Work out the finished part from the listing and answer in its coordinate system (mm). Face numbers are marked on the shaded views. A direction names the side the tool comes from. Round coordinates to 2 decimals unless told otherwise and drop trailing zeros. Loops run counter-clockwise (first coordinate to the right, second up) from the corner with the lowest first, then second, coordinate; pieces in that order, holes last. Notation, with made-up numbers: M -3.75,21.5 L 38.25,21.5 A17 ccw 38.25,41.5 Z; hole C 5,-10.5 d8. An arc over 180 degrees is marked long. One line per item, written item: value.
```python
from build123d import *

# Parameters (mm, degrees)
F0_W     = 76.2
F0_H     = 50.8
F0_R     = 12.7
F1_DEPTH = 12.7
F2_W     = 6.35
F2_H     = 50.8
F3_DEPTH = 2.54
F5_DEPTH = 50.801
F6_R     = 4.445
F7_DEPTH = 12.7


with BuildPart() as f1:
    # F0 (on Front) → F1 (new body)
    with BuildSketch(Plane.XZ):
        Rectangle(F0_W, F0_H)
        Circle(F0_R, mode=Mode.SUBTRACT)
    extrude(amount=F1_DEPTH)

    # F2 (on face) → F3 (cut)
    with BuildSketch(Plane.XZ.offset(12.7)):
        with Locations((-32.385, 0)):
            Rectangle(F2_W, F2_H)
        with BuildLine():
            Line((6.35, 25.4), (-6.35, 25.4))
            Line((-6.35, 25.4), (-6.35, 10.9985226281))
            ThreePointArc((-6.35, 10.9985226281), (0, 12.7), (6.35, 10.9985226281))
            Line((6.35, 10.9985226281), (6.35, 25.4))
        make_face()
        with BuildLine():
            Line((-6.35, -10.9985226281), (-6.35, -25.4))
            Line((-6.35, -25.4), (6.35, -25.4))
            Line((6.35, -25.4), (6.35, -10.9985226281))
            ThreePointArc((6.35, -10.9985226281), (0, -12.7), (-6.35, -10.9985226281))
        make_face()
    extrude(amount=-F3_DEPTH, mode=Mode.SUBTRACT)

    # F4 (on face) → F5 (cut, through all)
    with BuildSketch(Plane(origin=(0, 0, -25.4), x_dir=(1, 0, 0), z_dir=(0, 0, -1))):
        Polygon((31.75, 12.7), (19.05, 12.7), (16.1170606325, 7.62), (34.6829393675, 7.62), align=None)
    extrude(amount=-F5_DEPTH, mode=Mode.SUBTRACT)

    # F6 (on face) → F7 (join)
    with BuildSketch(Plane.YZ.offset(38.1)):
        with Locations((-6.35, 0)):
            Circle(F6_R)
    extrude(amount=F7_DEPTH)


solid = f1.part
```
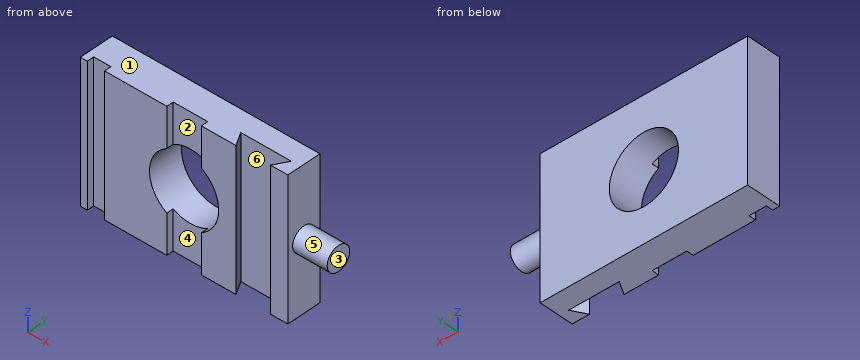
1) The mould has two halves that part along X. Classify the marked faces 3, 4, 5 and 6: +X half, -X half, draft (parallel to the pull), parting line (faces both ways), or undercut.
Check values:
face 3: +X half
face 4: undercut
face 5: draft
face 6: undercut
2) Find the intervals of material crossed by probe 1 along Z at (x, y) = (0, -10); probe 2 along X at (y, z) = (-4.75, 0); probe 3 along X at (y, z) = (-8.5, 1.5), in increasing order. Write a range as from..to.
Check values:
probe 1: -25.4..-12.7, 12.7..25.4
probe 2: -38.1..-12.7, 12.7..50.8
probe 3: -38.1..-12.61, 12.61..16.63, 34.17..50.8
3) Find section A-A (z = 0). Give the vertices of the cut face in (x, y) (3 decimals), then the cut area to 3 significant figures.
Check values:
outline: M -38.1,-12.7 L -35.56,-12.7 L -35.56,-10.16 L -29.21,-10.16 L -29.21,-12.7 L -12.7,-12.7 L -12.7,0 L -38.1,0 Z; M 12.7,-12.7 L 19.05,-12.7 L 16.117,-7.62 L 34.683,-7.62 L 31.75,-12.7 L 38.1,-12.7 L 38.1,-10.795 L 50.8,-10.795 L 50.8,-1.905 L 38.1,-1.905 L 38.1,0 L 12.7,0 Z
area: 663 mm2
4) Find section D-D (z = 17.5). Give the vertices of the cut face in (x, y).
Check values:
outline: M -38.1,-12.7 L -35.56,-12.7 L -35.56,-10.16 L -29.21,-10.16 L -29.21,-12.7 L -6.35,-12.7 L -6.35,-10.16 L 6.35,-10.16 L 6.35,-12.7 L 19.05,-12.7 L 16.12,-7.62 L 34.68,-7.62 L 31.75,-12.7 L 38.1,-12.7 L 38.1,0 L -38.1,0 Z
5) Find section B-B (x = 0). Give the vertices of the cut face in (y, z), then the cut area to 3 significant figures.
Check values:
outline: M -10.16,-25.4 L 0,-25.4 L 0,-12.7 L -10.16,-12.7 Z; M -10.16,12.7 L 0,12.7 L 0,25.4 L -10.16,25.4 Z
area: 258 mm2
6) For the marked faces 1 and 2, determine the directions among +Z, -Z, +X, -X, +Y, -Y from which every point of the face is accessible in a straight line to the end or side of a thin tool.
Check values:
face 1: +Z, +X, -X, +Y, -Y
face 2: +Z, -Z, -Y
7) Each of these flat-tipped pins is pushed along its axis until it touches: pin 1 (2 mm diameter, centred on y = -11, z = 16, fed in from +X); pin 2 (1.9 mm diameter, centred on x = -34, z = -12.5, fed in from -Y); pin 3 (5 mm diameter, centred on x = -0.5, z = 9, fed in from -Y). Where does it stop, or does it pass through?
Check values:
pin 1: x = 38.1
pin 2: y = -10.16
pin 3: through
8) Find section C-C (y = -6.35). Give the vertices of the cut face in (x, z) (3 decimals), then the cut area to 3 significant figures.
Check values:
outline: M -38.1,-25.4 L 38.1,-25.4 L 38.1,-4.445 L 50.8,-4.445 L 50.8,4.445 L 38.1,4.445 L 38.1,25.4 L -38.1,25.4 Z; hole C 0,0 d25.4
area: 3,480 mm2
